from build123d import *

# Parameters (mm, degrees)
SKETCH1_W                 = 108
SKETCH1_H                 = 207
BOSS_EXTRUDE1_DEPTH       = 2
SKETCH2_W                 = 100
SKETCH2_H                 = 199
BOSS_EXTRUDE2_DEPTH       = 2
CHAMFER1_SIZE             = 5
FILLET1_R                 = 5
F_3_0MM_DOWEL_HOLE1_D     = 3
F_3_0MM_DOWEL_HOLE1_DEPTH = 17.29
F_3_0MM_DOWEL_HOLE1_TIP   = 0.901290929
CHAMFER2_SIZE             = 1


with BuildPart() as part:
    # Sketch1 → Boss-Extrude1 (new body)
    with BuildSketch(Plane(origin=(0, 0, 0), x_dir=(1, 0, 0), z_dir=(0, 1, 0))):
        Rectangle(SKETCH1_W, SKETCH1_H)
    extrude(amount=BOSS_EXTRUDE1_DEPTH)

    # Sketch2 → Boss-Extrude2 (add)
    with BuildSketch(Plane(origin=(0, 2, 0), x_dir=(1, 0, 0), z_dir=(0, 1, 0))):
        Rectangle(SKETCH2_W, SKETCH2_H)
    extrude(amount=BOSS_EXTRUDE2_DEPTH)

    # Chamfer1
    chamfer1_edges = [part.edges().sort_by_distance(p)[0] for p in [
        (50, 3, 99.5),
        (50, 3, -99.5),
        (-50, 3, -99.5),
        (-50, 3, 99.5),
    ]]
    chamfer(chamfer1_edges, length=CHAMFER1_SIZE)

    # Fillet1
    fillet1_edges = [part.edges().sort_by_distance(p)[0] for p in [
        (-50, 3, 94.5),
        (-50, 3, -94.5),
        (45, 3, -99.5),
        (-45, 3, -99.5),
        (50, 3, 94.5),
        (50, 3, -94.5),
        (45, 3, 99.5),
        (-45, 3, 99.5),
        (54, 1, 103.5),
        (-54, 1, 103.5),
        (-54, 1, -103.5),
        (54, 1, -103.5),
    ]]
    fillet(fillet1_edges, radius=FILLET1_R)

    # Ø3.0mm Dowel Hole1
    with Locations(Plane(origin=(0, 0, 0), x_dir=(-1, 0, 0), z_dir=(0, -1, 0))):
        with Locations((-50, 99.5), (50, 99.5), (50, -99.5), (-50, -99.5)):
            Hole(F_3_0MM_DOWEL_HOLE1_D / 2, depth=F_3_0MM_DOWEL_HOLE1_DEPTH)
            with Locations((0, 0, -(F_3_0MM_DOWEL_HOLE1_DEPTH + F_3_0MM_DOWEL_HOLE1_TIP / 2))):  # 118° drill point
                Cone(0, F_3_0MM_DOWEL_HOLE1_D / 2, F_3_0MM_DOWEL_HOLE1_TIP, mode=Mode.SUBTRACT)

    # Chamfer2
    chamfer2_edges = [part.edges().sort_by_distance(p)[0] for p in [
        (0, 0, 103.5),
        (54, 0, 0),
        (-54, 0, 0),
        (0, 0, -103.5),
        (-52.535533906, 0, -102.035533906),
        (52.535533906, 0, -102.035533906),
        (52.535533906, 0, 102.035533906),
        (-52.535533906, 0, 102.035533906),
    ]]
    chamfer(chamfer2_edges, length=CHAMFER2_SIZE)


solid = part.part
CAD build for the part. Positions are in the model's coordinates, mm. Coordinates: 2 decimals unless noted, no trailing zeros. Order: outer loops, then holes, each group sorted by start corner. A loop starts at its lowest first (then second) coordinate and runs counter-clockwise, first axis right, second up.
Item 1: Band-saw the part on C-C on x = -25. List the corners of the cut face in (y, z).
Check sheet entries:
outline: (0, -102.5) - (1, -103.5) - (2, -103.5) - (2, -99.5) - (4, -99.5) - (4, 99.5) - (2, 99.5) - (2, 103.5) - (1, 103.5) - (0, 102.5) - close
Item 2: Drill centre lines: L1, parallel to X at y = 1, z = 99.5; L2, parallel to Z at x = 50, y = 0.75; L3, parallel to Z at x = 50, y = 0.6. Where is each one in solid material? Low to high.
Check sheet entries:
L1: x = -53.9 to -51.5, -48.5 to 48.5, 51.5 to 53.9
L2: z = -103.14 to -101, -98 to 98, 101 to 103.14
L3: z = -102.99 to -101, -98 to 98, 101 to 102.99
Item 3: Band-saw the part on B-B on y = 3.2. List the corners of the cut face in (x, z).
Check sheet entries:
outline: (-50, -92.43) arc R5 ccw to (-48.54, -95.96) - (-46.46, -98.04) arc R5 ccw to (-42.93, -99.5) - (42.93, -99.5) arc R5 ccw to (46.46, -98.04) - (48.54, -95.96) arc R5 ccw to (50, -92.43) - (50, 92.43) arc R5 ccw to (48.54, 95.96) - (46.46, 98.04) arc R5 ccw to (42.93, 99.5) - (-42.93, 99.5) arc R5 ccw to (-46.46, 98.04) - (-48.54, 95.96) arc R5 ccw to (-50, 92.43) - close
Item 4: Band-saw the part on A-A on z = -13. List the corners of the cut face in (x, y), plus the area to 3 significant figures.
Check sheet entries:
outline: (-54, 1) - (-53, 0) - (53, 0) - (54, 1) - (54, 2) - (50, 2) - (50, 4) - (-50, 4) - (-50, 2) - (-54, 2) - close
area: 415 mm2
Item 5: Pin check, flat tips, straight feed: pin 1 Ø3.5 at (x, z) = (50, 99.5) entering from +Y; pin 2 Ø1.8 at (x, z) = (-50, 99.5) entering from +Y; pin 3 Ø2 at (x, y) = (-3, 2.5) entering from -Z; pin 4 Ø0.6 at (y, z) = (3.5, -45) entering from +X. Stop position of each tip, or through.
Check sheet entries:
pin 1: stops at y = 2
pin 2: passes through
pin 3: stops at z = -103.5
pin 4: stops at x = 50
